Could you check a few things on this model? Use its own coordinates, in mm. Face numbers are marked on the shaded views. Coordinates: 2 decimals unless noted, no trailing zeros. Order: outer loops, then holes, each group sorted by start corner. A loop starts at its lowest first (then second) coordinate and runs counter-clockwise, first axis right, second up. Notation, with made-up numbers: (31.5, -16.5) -> (74.5, -16.5) arc R17 ccw to (74.5, -5.5) -> close; hole circle Ø6 at (-4, 27.25). An arc over 180 degrees is marked (long way). Return JSON: item names as keys, results as strings. Group by question number.
from build123d import *

# Parameters (mm, degrees)
F0_W     = 35
F0_H     = 70
F1_DEPTH = 3
F3_DEPTH = 3
F5_DEPTH = 3


# Not quite as in the source:
# - a feature names something its author has since deleted; it is built from what else it names


with BuildPart() as f1:
    # F0 (on Top) → F1 (new body)
    with BuildSketch(Plane.XY):
        with Locations((-17.5, 35)):
            Rectangle(F0_W, F0_H)
    extrude(amount=F1_DEPTH)

    # F2 (on face) → F3 (join)
    with BuildSketch(Plane(origin=(-35, 0, 0), x_dir=(0, -1, 0), z_dir=(-1, 0, 0))):
        Polygon((-35, 86.622338891), (-3, 59.4277828932), (-3, 62.8054440022), (-33.0127427803, 88.3111694455), align=None)
        Polygon((-67, 62.8054440022), (-67, 59.4277828932), (-35, 86.622338891), (-36.9872572197, 88.3111694455), align=None)
        Polygon((-70, 93), (-70, 90), (-67, 90), (-38.9745144394, 90), (-35, 90), (-35, 93), align=None)
        Polygon((0, 93), (-35, 93), (-35, 90), (-31.0254855606, 90), (-3, 90), (0, 90), align=None)
        Polygon((-35, 90), (-33.0127427803, 88.3111694455), (-31.0254855606, 90), align=None)
        Polygon((-36.9872572197, 88.3111694455), (-35, 86.622338891), (-33.0127427803, 88.3111694455), (-35, 90), align=None)
        Polygon((-35, 90), (-38.9745144394, 90), (-36.9872572197, 88.3111694455), align=None)
        Polygon((-70, 90), (-70, 3), (-67, 3), (-67, 59.4277828932), (-67, 62.8054440022), (-67, 90), align=None)
        Polygon((-3, 59.4277828932), (-3, 3), (0, 3), (0, 90), (-3, 90), (-3, 62.8054440022), align=None)
    extrude(amount=-F3_DEPTH)

    # F4 (on face) → F5 (join)
    with BuildSketch(Plane.XY.offset(93)):
        with BuildLine():
            Line((-32, 70), (-32, 0))
            Line((-32, 0), (0, 0))
            Line((0, 0), (0, 32))
            ThreePointArc((0, 32), (-1.7320508076, 32.5505102572), (-2.8284271247, 34))
            ThreePointArc((-2.8284271247, 34), (-3, 35), (-2.8284271247, 36))
            ThreePointArc((-2.8284271247, 36), (-1.7320508076, 37.4494897428), (0, 38))
            Line((0, 38), (0, 70))
            Line((0, 70), (-32, 70))
        make_face()
        with BuildLine():
            Line((-2.8284271247, 34), (0, 34))
            Line((0, 34), (0, 36))
            Line((0, 36), (-2.8284271247, 36))
            ThreePointArc((-2.8284271247, 36), (-3, 35), (-2.8284271247, 34))
        make_face()
    extrude(amount=-F5_DEPTH)

    # F6: F1 across plane


with BuildPart() as f1_1:
    add(f1.part)
    add(f1.part.mirror(Plane.YZ))


solid = f1_1.part
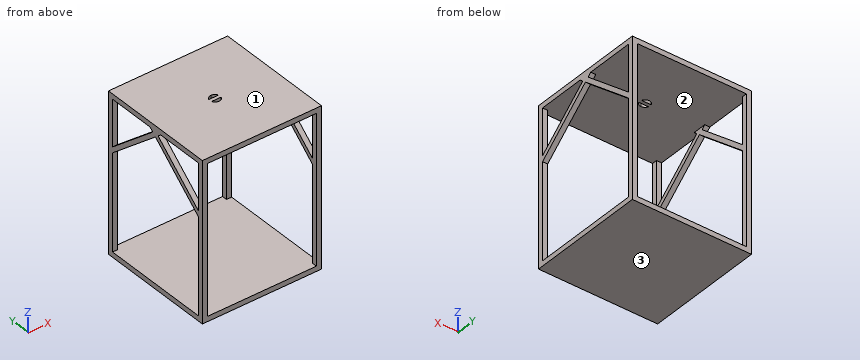
Q1. I want a section at A-A on x = -24. Please give me the cut outline in (y, z).
Q2. I need wall thicknesses on line 1 along Z through (x, y) = (-18.5, 64.5); line 2 along X through (y, z) = (26, 82). Which ranges of each line are inside material? Lowest first, please. Write a range as from..to.
Q3. I want a section at C-C on y = 47. Please give me the cut outline in (x, z).
Q4. I want a section at D-D on z = 69. State how many separate pieces and enclosed holes the cut face has, and give its area (3 significant figures).
Q5. I want a section at B-B on z = 53. Please give me the cut outline in (x, y).
Q6. We'd pull the mould along Z, two halves only. Please class the marked faces 1, 2 and 3: pulls with the +Z half, pulls with the -Z half, needs draft (parallel to the pull), parting line crosses it, or undercut.
Response values:
{
 "1": {"outline": "(0, 0) -> (70, 0) -> (70, 3) -> (0, 3) -> close; (0, 90) -> (70, 90) -> (70, 93) -> (0, 93) -> close"},
 "2": {"line 1": "z = 0..3, 90..93", "line 2": "x = -35..-32, 32..35"},
 "3": {"outline": "(-35, 0) -> (35, 0) -> (35, 3) -> (-35, 3) -> close; (-35, 76.42) -> (-32, 76.42) -> (-32, 79.8) -> (-35, 79.8) -> close; (-35, 90) -> (35, 90) -> (35, 93) -> (-35, 93) -> close; (32, 76.42) -> (35, 76.42) -> (35, 79.8) -> (32, 79.8) -> close"},
 "4": {"separate pieces": "8", "enclosed holes": "0", "area": "83.7 mm²"},
 "5": {"outline": "(-35, 0) -> (-32, 0) -> (-32, 3) -> (-35, 3) -> close; (-35, 67) -> (-32, 67) -> (-32, 70) -> (-35, 70) -> close; (32, 0) -> (35, 0) -> (35, 3) -> (32, 3) -> close; (32, 67) -> (35, 67) -> (35, 70) -> (32, 70) -> close"},
 "6": {"face 1": "pulls with the +Z half", "face 2": "undercut", "face 3": "pulls with the -Z half"}
}
